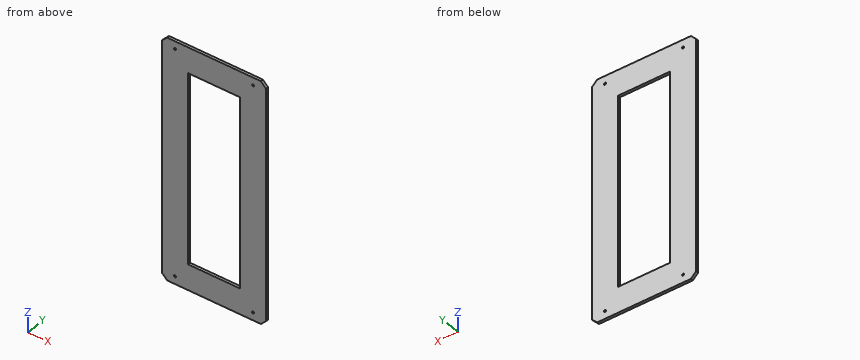
```python
from build123d import *

# Parameters (mm, degrees)
F0_W     = 200
F0_H     = 470
F0_W_2   = 100
F0_H_2   = 370
F1_DEPTH = 5
F2_SIZE  = 10
F4_D     = 4
F4_DEPTH = 8


with BuildPart() as f1:
    # F0 (on Front) → F1 (new body)
    with BuildSketch(Plane.XZ):
        Rectangle(F0_W, F0_H)
        Rectangle(F0_W_2, F0_H_2, mode=Mode.SUBTRACT)
    extrude(amount=F1_DEPTH)

    # F2
    f2_edges = [f1.edges().sort_by_distance(p)[0] for p in [
        (-100, -2.5, 235),
        (100, -2.5, 235),
        (100, -2.5, -235),
        (-100, -2.5, -235),
    ]]
    chamfer(f2_edges, length=F2_SIZE)

    # F4
    with Locations(Plane.XZ.offset(5)):
        with Locations((-75, 220), (75, 220), (-75, -220), (75, -220)):
            Hole(F4_D / 2, depth=F4_DEPTH)


solid = f1.part
```
CAD build for the part. Positions are in the model's coordinates, mm. Round coordinates to 2 decimals unless told otherwise and drop trailing zeros. Loops run counter-clockwise (first coordinate to the right, second up) from the corner with the lowest first, then second, coordinate; pieces in that order, holes last. Notation, with made-up numbers: M 62.5,21 L 110.5,21 A12 cw 110.5,44 Z; hole C 51,83 d8. An arc over 180 degrees is marked long. Return JSON: item names as keys, results as strings. Group by question number.
(1) Wall check: probe 1 along X at (y, z) = (-1.6, 220); probe 2 along Z at (x, y) = (-75, -1.9); probe 3 along Z at (x, y) = (32.5, -3.7). Give the ranges that are in metal, low to high. Write a range as [from, to].
(2) Saw through at B-B, the plane x = 44.5. List the corners of the cut face in (y, z), and give its area (3 significant figures).
(3) Saw through at A-A, the plane z = -155.5. List the corners of the cut face in (x, y).
(4) Saw through at C-C, the plane y = -1.7. List the corners of the cut face in (x, z).
Answer list:
{
 "1": {"probe 1": "[-100, -77], [-73, 73], [77, 100]", "probe 2": "[-235, -222], [-218, 218], [222, 235]", "probe 3": "[-235, -185], [185, 235]"},
 "2": {"outline": "M -5,-235 L 0,-235 L 0,-185 L -5,-185 Z; M -5,185 L 0,185 L 0,235 L -5,235 Z", "area": "500 mm2"},
 "3": {"outline": "M -100,-5 L -50,-5 L -50,0 L -100,0 Z; M 50,-5 L 100,-5 L 100,0 L 50,0 Z"},
 "4": {"outline": "M -100,-225 L -90,-235 L 90,-235 L 100,-225 L 100,225 L 90,235 L -90,235 L -100,225 Z; hole C -75,-220 d4; hole C -75,220 d4; hole M -50,-185 L 50,-185 L 50,185 L -50,185 Z; hole C 75,-220 d4; hole C 75,220 d4"}
}
